Read the model definition and answer for the solid it produces. Units are mm, in the model's axes. Face numbers are marked on the shaded views. A direction names the side the tool comes from. Coordinates: 2 decimals unless noted, no trailing zeros. Loops run counter-clockwise (first coordinate to the right, second up) from the corner with the lowest first, then second, coordinate; pieces in that order, holes last. Notation, with made-up numbers: (28.5, 39.5) -> (85.5, 39.5) arc R31 ccw to (85.5, 72.5) -> close; hole circle Ø8 at (82.25, -4.5). An arc over 180 degrees is marked (long way). Answer in a Markdown table with one row per item.
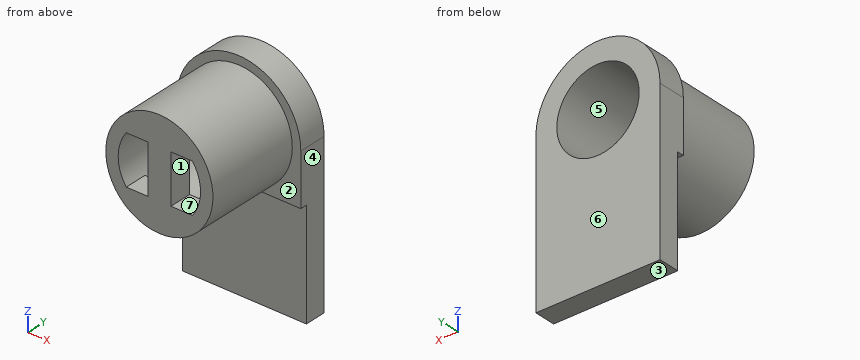
```python
from build123d import *

# Parameters (mm, degrees)
SKETCH1_R           = 4.75
SKETCH1_R_2         = 3.65
BOSS_EXTRUDE1_DEPTH = 2
SKETCH2_R           = 4.75
SKETCH2_R_2         = 3.65
BOSS_EXTRUDE2_DEPTH = 6.5
SKETCH3_R           = 3.65
BOSS_EXTRUDE3_DEPTH = 2.5
CUT_EXTRUDE1_START  = -1.9
SKETCH5_W           = 11
SKETCH5_H           = 9.490844779
CUT_EXTRUDE1_DEPTH  = 1


with BuildPart() as part:
    # Sketch1 → Boss-Extrude1 (new body)
    # profile 1 of 9: a face of its own
    with BuildSketch(Plane(origin=(0, 0, 0), x_dir=(1, 0, 0), z_dir=(0, 1, 0))):
        with Locations(Location((0, 0, 0), (0, 0, 270))):
            Circle(SKETCH1_R)
        Circle(SKETCH1_R_2, mode=Mode.SUBTRACT)
    # profile 2 of 9: a face of its own
    with BuildSketch(Plane(origin=(0, 0, 0), x_dir=(1, 0, 0), z_dir=(0, 1, 0))):
        with BuildLine():
            Line((1.028169014, 3.502194809), (1.028169014, 2.171577767))
            Line((1.028169014, 2.171577767), (2.9337263, 2.171577767))
            ThreePointArc((2.9337263, 2.171577767), (2.089686351, 2.992609389), (1.028169014, 3.502194809))
        make_face()
    # profile 3 of 9: a face of its own
    with BuildSketch(Plane(origin=(0, 0, 0), x_dir=(1, 0, 0), z_dir=(0, 1, 0))):
        with BuildLine():
            Line((-1.028169014, 2.171577767), (1.028169014, 2.171577767))
            Line((1.028169014, 2.171577767), (1.028169014, 3.502194809))
            ThreePointArc((1.028169014, 3.502194809), (0, 3.65), (-1.028169014, 3.502194809))
            Line((-1.028169014, 3.502194809), (-1.028169014, 2.171577767))
        make_face()
    # profile 4 of 9: a face of its own
    with BuildSketch(Plane(origin=(0, 0, 0), x_dir=(1, 0, 0), z_dir=(0, 1, 0))):
        with BuildLine():
            Line((-2.9337263, 2.171577767), (-1.028169014, 2.171577767))
            Line((-1.028169014, 2.171577767), (-1.028169014, 3.502194809))
            ThreePointArc((-1.028169014, 3.502194809), (-2.089686351, 2.992609389), (-2.9337263, 2.171577767))
        make_face()
    # profile 5 of 9: a face of its own
    with BuildSketch(Plane(origin=(0, 0, 0), x_dir=(1, 0, 0), z_dir=(0, 1, 0))):
        Polygon((-1.028169014, 0), (0, 0), (1.028169014, 0), (1.028169014, 2.171577767), (-1.028169014, 2.171577767), align=None)
    # profile 6 of 9: a face of its own
    with BuildSketch(Plane(origin=(0, 0, 0), x_dir=(1, 0, 0), z_dir=(0, 1, 0))):
        Polygon((1.028169014, 0), (0, 0), (-1.028169014, 0), (-1.028169014, -2.171577767), (1.028169014, -2.171577767), align=None)
    # profile 7 of 9: a face of its own
    with BuildSketch(Plane(origin=(0, 0, 0), x_dir=(1, 0, 0), z_dir=(0, 1, 0))):
        with BuildLine():
            Line((1.028169014, -3.502194809), (1.028169014, -2.171577767))
            Line((1.028169014, -2.171577767), (-1.028169014, -2.171577767))
            Line((-1.028169014, -2.171577767), (-1.028169014, -3.502194809))
            ThreePointArc((-1.028169014, -3.502194809), (0, -3.65), (1.028169014, -3.502194809))
        make_face()
    # profile 8 of 9: a face of its own
    with BuildSketch(Plane(origin=(0, 0, 0), x_dir=(1, 0, 0), z_dir=(0, 1, 0))):
        with BuildLine():
            Line((-1.028169014, -3.502194809), (-1.028169014, -2.171577767))
            Line((-1.028169014, -2.171577767), (-2.9337263, -2.171577767))
            ThreePointArc((-2.9337263, -2.171577767), (-2.089686351, -2.992609389), (-1.028169014, -3.502194809))
        make_face()
    # profile 9 of 9: a face of its own
    with BuildSketch(Plane(origin=(0, 0, 0), x_dir=(1, 0, 0), z_dir=(0, 1, 0))):
        with BuildLine():
            Line((2.9337263, -2.171577767), (1.028169014, -2.171577767))
            Line((1.028169014, -2.171577767), (1.028169014, -3.502194809))
            ThreePointArc((1.028169014, -3.502194809), (2.089686351, -2.992609389), (2.9337263, -2.171577767))
        make_face()
    extrude(amount=BOSS_EXTRUDE1_DEPTH)

    # Sketch2 → Boss-Extrude2 (add)
    with BuildSketch(Plane(origin=(0, 2, 0), x_dir=(1, 0, 0), z_dir=(0, 1, 0))):
        with Locations(Location((0, 0, 0), (0, 0, 270))):
            Circle(SKETCH2_R)
        with Locations(Location((0, 0, 0), (0, 0, 36.509268316))):
            Circle(SKETCH2_R_2, mode=Mode.SUBTRACT)
    extrude(amount=BOSS_EXTRUDE2_DEPTH)

    # Sketch3 → Boss-Extrude3 (add)
    with BuildSketch(Plane(origin=(0, 8.5, 0), x_dir=(1, 0, 0), z_dir=(0, 1, 0))):
        with BuildLine():
            ThreePointArc((-5.5, 0), (0, -5.5), (5.5, 0))
            Line((5.5, 0), (5.5, 14.1))
            Line((5.5, 14.1), (-5.5, 14.1))
            Line((-5.5, 14.1), (-5.5, 0))
        make_face()
        with Locations(Location((0, 0, 0), (0, 0, 36.509268316))):
            Circle(SKETCH3_R, mode=Mode.SUBTRACT)
    extrude(amount=BOSS_EXTRUDE3_DEPTH)

    # Sketch5 → Cut-Extrude1 (cut)
    with BuildSketch(Plane(origin=(0, 11, 0), x_dir=(1, 0, 0), z_dir=(0, 1, 0)).offset(CUT_EXTRUDE1_START)):
        with Locations((0, 9.354577611)):
            Rectangle(SKETCH5_W, SKETCH5_H)
    extrude(amount=-CUT_EXTRUDE1_DEPTH, mode=Mode.SUBTRACT)


solid = part.part
```
1. A cutting plane is placed at A-A on y = 8.75. Give the vertices of the cut face in (x, z).
A:
| item | result |
|---|---|
| outline | (-5.5, -4.61) -> (5.5, -4.61) -> (5.5, 0) arc R5.5 ccw to (-5.5, 0) -> close; hole circle Ø7.3 at (0, 0) |
2. A cutting plane is placed at D-D on x = 1.5. Give the vertices of the cut face in (y, z), and give its area (3 significant figures).
A:
| item | result |
|---|---|
| outline | (0, -4.51) -> (8.5, -4.51) -> (8.5, -4.61) -> (9.1, -4.61) -> (9.1, -14.1) -> (11, -14.1) -> (11, -3.33) -> (2, -3.33) -> (2, -2.17) -> (0, -2.17) -> close; (0, 2.17) -> (2, 2.17) -> (2, 3.33) -> (11, 3.33) -> (11, 5.29) -> (8.5, 5.29) -> (8.5, 4.51) -> (0, 4.51) -> close |
| area | 50.8 mm2 |
3. A cutting plane is placed at B-B on z = -1.5. Give the vertices of the cut face in (x, y).
A:
| item | result |
|---|---|
| outline | (-5.5, 8.5) -> (-4.51, 8.5) -> (-4.51, 0) -> (-3.33, 0) -> (-3.33, 11) -> (-5.5, 11) -> close; (-1.03, 0) -> (1.03, 0) -> (1.03, 2) -> (-1.03, 2) -> close; (3.33, 0) -> (4.51, 0) -> (4.51, 8.5) -> (5.5, 8.5) -> (5.5, 11) -> (3.33, 11) -> close |
4. The mould has two halves that part along X. Classify the marked faces 4, 5, 6 and 7: pulls with the +X half, pulls with the -X half, needs draft (parallel to the pull), parting line crosses it, or undercut.
A:
| item | result |
|---|---|
| face 4 | pulls with the +X half |
| face 5 | undercut |
| face 6 | needs draft |
| face 7 | undercut |
5. Find the intervals of material crossed by probe 1 along X at (y, z) = (3.5, 0); probe 2 along Z at (x, y) = (0, 8.75), in increasing order.
A:
| item | result |
|---|---|
| probe 1 | x = -4.75 to -3.65, 3.65 to 4.75 |
| probe 2 | z = -4.61 to -3.65, 3.65 to 5.5 |
6. A cutting plane is placed at C-C on x = 0. Give the vertices of the cut face in (y, z), and give its area (3 significant figures).
A:
| item | result |
|---|---|
| outline | (0, -4.75) -> (8.1, -4.75) -> (8.1, -4.61) -> (9.1, -4.61) -> (9.1, -14.1) -> (11, -14.1) -> (11, -3.65) -> (2, -3.65) -> (2, 3.65) -> (11, 3.65) -> (11, 5.5) -> (8.5, 5.5) -> (8.5, 4.75) -> (0, 4.75) -> close |
| area | 58.3 mm2 |
7. A tool of negligible diameter and unlimited length cuts with its end or side. For the marked faces 1, 2 and 3, from which of +Z, -Z, +X, -X, +Y, -Y can it reach the whole face along a straight path? Write none if from no direction.
A:
| item | result |
|---|---|
| face 1 | +Y, -Y |
| face 2 | -Y |
| face 3 | -Z, +X, -X, +Y, -Y |
8. Given pin 1 Ø1.5 at (x, y) = (-2, 1) entering from -Z; pin 2 Ø1 at (x, y) = (-2, 1) entering from +Z; pin 3 Ø6 at (x, y) = (2.5, 1) entering from -Z, each flat-ended and moving along its own axis, determine where each tip first touches the part or whether it passes through.
A:
| item | result |
|---|---|
| pin 1 | stops at z = -4.58 |
| pin 2 | stops at z = 4.51 |
| pin 3 | stops at z = -4.75 |
